Read the model definition and answer for the solid it produces. Units are mm, in the model's axes. Face numbers are marked on the shaded views. A direction names the side the tool comes from. Coordinates: 2 decimals unless noted, no trailing zeros. Order: outer loops, then holes, each group sorted by start corner. A loop starts at its lowest first (then second) coordinate and runs counter-clockwise, first axis right, second up. Notation, with made-up numbers: (69.25, 60) -> (126.25, 60) arc R24 ccw to (126.25, 71) -> close; hole circle Ø5 at (19, -0.75). An arc over 180 degrees is marked (long way). Use CSV: the item, a comma, the result in double quotes.
Solid Edge part; units mm, degrees
sketch "Sketch1" plane through (0, 0, 0) normal (0, -1, 0) x (1, 0, 0)
  line L0 (0, 0) -> (-30, 0)
  line L1 (-30, 0) -> (-30, -4)
  line L2 (0, -4) -> (-30, -4)
  line L3 (19.2132, -23.2132) -> (0, -4)
  line L4 (21.2132, -21.2132) -> (19.2132, -23.2132)
  line L5 (0, 0) -> (21.2132, -21.2132)
  dimension "D1" = 30
extrude "Protrusion1" add sketch "Sketch1" along normal mid plane 30
sketch "Sketch2" plane through (-15, 0, 0) normal (0, 0, 1) x (1, 0, 0)
  circle A0 centre (0.28, 0) radius 7.5
  dimension "D1" = 0.28
extrude "Cutout1" cut sketch "Sketch2" against normal up to surface (4 mm away)
sketch "Sketch3" plane through (10.6066, 0, -10.6066) normal (0.7071068, 0, 0.7071068) x (0.7071068, 0, -0.7071068)
  circle A0 centre (-0.28, 0) radius 7.5
  dimension "D1" = 0.28
extrude "Cutout2" cut sketch "Sketch3" against normal up to surface (2.8284 mm away)
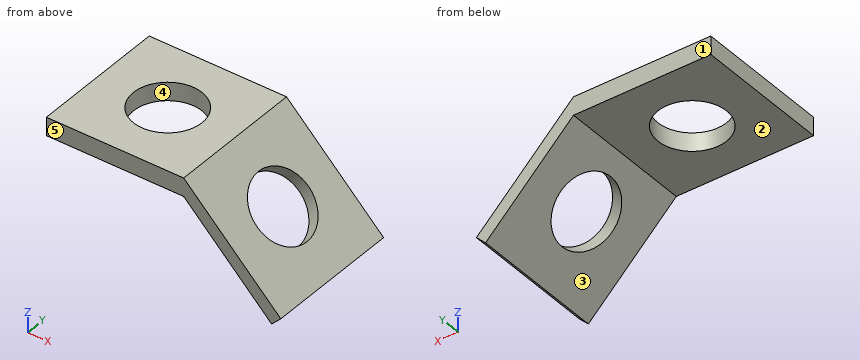
Item 1: The mould has two halves that part along Y. Classify the marked faces 3, 4 and 5: +Y half, -Y half, draft (parallel to the pull), parting line (faces both ways), or undercut.
Return value:
face 3,"draft"
face 4,"undercut"
face 5,"-Y half"
Item 2: Find section C-C, the plane z = -3.25. Give the vertices of the cut face in (x, y), then the cut area to 3 significant figures.
Return value:
outline,"(-30, -15) -> (3.25, -15) -> (3.25, 15) -> (-30, 15) -> close; hole circle Ø15 at (-14.72, 0)"
area,"821 mm^2"
Item 3: Find section D-D, the plane x = -21.5. Give the vertices of the cut face in (y, z).
Return value:
outline,"(-15, -4) -> (-3.21, -4) -> (-3.21, 0) -> (-15, 0) -> close; (3.21, -4) -> (15, -4) -> (15, 0) -> (3.21, 0) -> close"
Item 4: Straight lines are drawn through the part: line 1 along Y through (x, z) = (-14.72, -2.95); line 2 along Z through (x, y) = (-15.5, 11.25); line 3 along Z through (x, y) = (1, 12). For each, find the intervals that lie inside material, in ascending order.
Return value:
line 1,"y = -15 to -7.5, 7.5 to 15"
line 2,"z = -4 to 0"
line 3,"z = -5 to -1"
Item 5: Find section A-A, the plane x = -14.72. Give the vertices of the cut face in (y, z), then the cut area to 3 significant figures.
Return value:
outline,"(-15, -4) -> (-7.5, -4) -> (-7.5, 0) -> (-15, 0) -> close; (7.5, -4) -> (15, -4) -> (15, 0) -> (7.5, 0) -> close"
area,"60.0 mm^2"
Item 6: Each of these flat-tipped pins is pushed along its axis until it touches: P1, Ø1.5, axis at y = -9, z = -19.5, coming from the +X side; P2, Ø12, axis at x = -3.5, y = -3, coming from the +Z side; P3, Ø6, axis at y = 10, z = -11.5, coming from the +X side; P4, Ø8, axis at y = -9, z = -7.5, coming from the +X side. Where does it stop, or does it pass through?
Return value:
P1,"stops at x = 20.25"
P2,"stops at z = 0"
P3,"stops at x = 14.5"
P4,"stops at x = 11.5"
Item 7: Find section B-B, the plane y = -4.5. Give the vertices of the cut face in (x, z), then the cut area to 3 significant figures.
Return value:
outline,"(-30, -4) -> (-20.72, -4) -> (-20.72, 0) -> (-30, 0) -> close; (-8.72, -4) -> (0, -4) -> (4.17, -8.17) -> (6.17, -6.17) -> (0, 0) -> (-8.72, 0) -> close; (12.65, -16.65) -> (19.21, -23.21) -> (21.21, -21.21) -> (14.65, -14.65) -> close"
area,"119 mm^2"
Item 8: A tool of negligible diameter and unlimited length cuts with its end or side. For the marked faces 1 and 2, from which of +Z, -Z, +X, -X, +Y, -Y can it reach the whole face along a straight path? Write none if from no direction.
Return value:
face 1,"+Z, -Z, +X, -X, +Y"
face 2,"-Z, -X, +Y, -Y"
